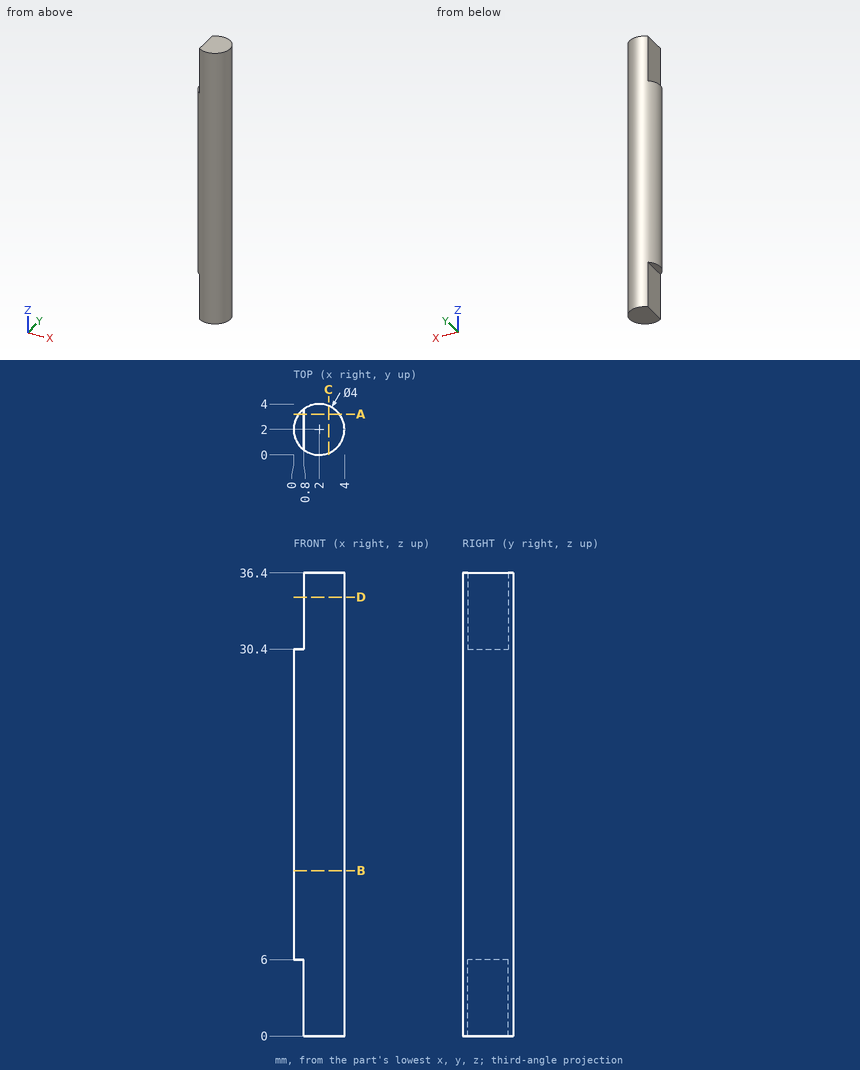
Here's the drawing with two shaded views (mm, measured from the low corner). I have some questions. Round coordinates to 2 decimals unless told otherwise and drop trailing zeros. Loops run counter-clockwise (first coordinate to the right, second up) from the corner with the lowest first, then second, coordinate; pieces in that order, holes last. Notation, with made-up numbers: M 40,0 L 65,0 A5 ccw 65,8 Z; hole C 0.25,23 d1. An arc over 180 degrees is marked long. Answer as a JSON object with one key per item and string values. Group by question number.
Q1. Imagine slicing it at B-B, the plane z = 13. Please give me the cut outline in (x, y).
Q2. Imagine slicing it at A-A, the plane y = 3.2. Please give me the cut outline in (x, z).
Q3. Please list where these lines run through material, in increasing order: L1, parallel to Z at x = 0.45, y = 2.7; L2, parallel to Y at x = 1.85, z = 3; L3, parallel to X at y = 2.1, z = 24.
Q4. Will these pins go through, and if not, where does the flat tip stop? pin 1 (1 mm diameter, centred on y = 2, z = 2, fed in from -X); pin 2 (1 mm diameter, centred on x = 0.5, z = 28.5, fed in from -Y).
Q5. Imagine slicing it at D-D, the plane z = 34.5. Please give me the cut outline in (x, y).
Q6. Imagine slicing it at C-C, the plane x = 2.75. Please give me the cut outline in (y, z).
Findings:
{
 "1": {"outline": "C 2,2 d4"},
 "2": {"outline": "M 0.4,6 L 0.8,6 L 0.8,0 L 3.6,0 L 3.6,36.4 L 0.8,36.4 L 0.8,30.4 L 0.4,30.4 Z"},
 "3": {"L1": "z = 6 to 30.4", "L2": "y = 0.01 to 3.99", "L3": "x = 0 to 4"},
 "4": {"pin 1": "stops at x = 0.8", "pin 2": "stops at y = 0.27"},
 "5": {"outline": "M 0.8,0.4 A2 ccw long 0.8,3.6 Z"},
 "6": {"outline": "M 0.15,0 L 3.85,0 L 3.85,36.4 L 0.15,36.4 Z"}
}
